Source: CAD feature listing. Evaluate the final solid. Frame: model axes, mm. A direction names the side the tool comes from. Give positions to 0.01 mm unless a question says otherwise; leave off trailing zeros. Order: outer loops, then holes, each group sorted by start corner. A loop starts at its lowest first (then second) coordinate and runs counter-clockwise, first axis right, second up.
Autodesk Inventor part; units mm, degrees
ref_plane "YZ Plane" through (0, 0, 0) normal (1, 0, 0) x (0, 1, 0)
ref_plane "XZ Plane" through (0, 0, 0) normal (0, 1, 0) x (-1, 0, 0)
ref_plane "XY Plane" through (0, 0, 0) normal (0, 0, 1) x (1, 0, 0)
sketch "Sketch1" plane through (0, 0, 0) normal (0, 1, 0) x (-1, 0, 0)
  circle A0 centre (0, 0) radius 55
  circle A1 centre (0, 0) radius 2.6
  dimension "d0" = 110
  dimension "d1" = 5.2
extrude "Extrusion1" add sketch "Sketch1" along normal blind 5
sketch "Sketch2" plane through (0, 5, 0) normal (0, 1, 0) x (1, 0, 0)
  point P0 (0, 0)
sketch "Sketch4" plane through (0, 5, 0) normal (0, 1, 0) x (1, 0, 0)
  circle A0 centre (0, 0) radius 21.9076
  circle A1 centre (0, 0) radius 35
  circle A2 centre (-35, 0) radius 15.2
  circle A3 centre (-17.5, -30.3109) radius 15.2
  circle A4 centre (17.5, -30.3109) radius 15.2
  circle A5 centre (35, 0) radius 15.2
  circle A6 centre (17.5, 30.3109) radius 15.2
  circle A7 centre (-17.5, 30.3109) radius 15.2
  circle A8 centre (-21.9076, 0) radius 5.15
  circle A9 centre (-15.491, -15.491) radius 5.15
  circle A10 centre (0, -21.9076) radius 5.15
  circle A11 centre (15.491, -15.491) radius 5.15
  circle A12 centre (21.9076, 0) radius 5.15
  circle A13 centre (15.491, 15.491) radius 5.15
  circle A14 centre (0, 21.9076) radius 5.15
  circle A15 centre (-15.491, 15.491) radius 5.15
  dimension "d13" = 70
  dimension "d8" = 30.4
  dimension "d11" = 360
  dimension "d14" = 10.3
  dimension "d17" = 360
extrude "Extrusion3" cut sketch "Sketch4" against normal blind 5 contours A0 A12 A5 | A0 A12 | A12 A5 A0 | A0 A5 A1 A12 | A0 A5 A12 | A5 A1 | A6 A13 A0 | A0 A13 A6 | A6 A0 A13 | A13 A0 A6 A14 A1 | A1 A6 | A4 A11 A0 | A0 A11 A4 | A4 A1 A10 A0 A11 | A11 A0 A4 | A4 A1 | A6 A14 | A7 A14 A0 A15 A1 | A1 A7 | A10 A4 | A3 A1 | A1 A3 A9 A0 A10 | A7 A14 | A10 A3 | A7 A15 A0 | A2 A0 A8 A1 | A1 A2 | A15 A0 A7 | A0 A9 A3 | A3 A0 A9 | A15 A7 A0 | A2 A8 A0 | A0 A3 A9 | A0 A8 A2 | A8 A2 A0 | A0 A8 picked at (11.9722, 17.0625) picked at (16.7139, 17.1312) picked at (8.2786, 19.0961) picked at (16.7139, -17.1312) picked at (11.9722, -17.0625) picked at (8.2786, -19.0961) picked at (-8.2786, 19.0961) picked at (-16.7226, 17.1255) picked at (-8.2786, -19.0961) picked at (-16.7226, -17.1255) picked at (-11.9722, 17.0625) picked at (-11.9722, -17.0625)
sketch "Sketch5" plane through (0, 5, 0) normal (0, 1, 0) x (1, 0, 0)
  point P0 (0, 0)
sketch "Sketch6" plane through (0, 0, 0) normal (0, -1, 0) x (1, 0, 0)
  circle A0 centre (0, 0) radius 55
extrude "Extrusion4" add sketch "Sketch6" along normal blind 0.5
sketch "Sketch7" plane through (0, 5, 0) normal (0, 1, 0) x (1, 0, 0)
  circle A0 centre (-35, 0) radius 15.2
  circle A1 centre (-35, 0) radius 12.5
  circle A2 centre (-17.5, -30.3109) radius 15.2
  circle A3 centre (-17.5, -30.3109) radius 12.5
  circle A4 centre (17.5, -30.3109) radius 15.2
  circle A5 centre (17.5, -30.3109) radius 12.5
  circle A6 centre (35, 0) radius 15.2
  circle A7 centre (35, 0) radius 12.5
  circle A8 centre (17.5, 30.3109) radius 15.2
  circle A9 centre (17.5, 30.3109) radius 12.5
  circle A10 centre (-17.5, 30.3109) radius 15.2
  circle A11 centre (-17.5, 30.3109) radius 12.5
  point P0 (0, 0)
  dimension "d23" = 25
  dimension "d24" = 25
  dimension "d25" = 25
  dimension "d26" = 25
  dimension "d27" = 25
  dimension "d28" = 25
extrude "Extrusion5" cut sketch "Sketch7" against normal blind 86.25 contours A1 | A3 | A5 | A7 | A9 | A11
sketch "Sketch8" plane through (0, 5, 0) normal (0, 1, 0) x (1, 0, 0)
  circle A0 centre (0, 0) radius 2.6
extrude "Extrusion6" cut sketch "Sketch8" against normal blind 86.25
sketch "Sketch9" plane through (0, 5, 0) normal (0, 1, 0) x (1, 0, 0)
  circle A0 centre (17.5, 30.3109) radius 15.2
  arc A1 (26.25, 15.1554) -> (0, 30.3109) centre (17.5, 30.3109) ccw
  circle A2 centre (35, 0) radius 15.2
  arc A3 (26.25, -15.1554) -> (26.25, 15.1554) centre (35, 0) ccw
  circle A4 centre (17.5, -30.3109) radius 15.2
  arc A5 (0, -30.3109) -> (26.25, -15.1554) centre (17.5, -30.3109) ccw
  circle A6 centre (-17.5, -30.3109) radius 15.2
  arc A7 (-26.25, -15.1554) -> (0, -30.3109) centre (-17.5, -30.3109) ccw
  circle A8 centre (-35, 0) radius 15.2
  arc A9 (-26.25, 15.1554) -> (-26.25, -15.1554) centre (-35, 0) ccw
  circle A10 centre (-17.5, 30.3109) radius 15.2
  arc A11 (0, 30.3109) -> (-26.25, 15.1554) centre (-17.5, 30.3109) ccw
  circle A12 centre (0, 0) radius 2.6
  circle A13 centre (0, 0) radius 65.8368
  dimension "d33" = 35
  dimension "d34" = 35
  dimension "d35" = 35
  dimension "d36" = 35
  dimension "d37" = 35
  dimension "d38" = 35
  dimension "d39" = 131.6736
extrude "Extrusion7" cut sketch "Sketch9" against normal blind 86.25 contours A13
properties part number "generator 12smaller"
1) Section query C-C, the plane y = 3.85. Return the cut outline in (x, z).
Report:
outline: (-26.25, -15.16) arc R17.5 ccw (long way) to (0, -30.31) arc R17.5 ccw (long way) to (26.25, -15.16) arc R17.5 ccw (long way) to (26.25, 15.16) arc R17.5 ccw (long way) to (0, 30.31) arc R17.5 ccw (long way) to (-26.25, 15.16) arc R17.5 ccw (long way) to start; hole circle Ø30.4 at (-35, 0); hole circle Ø30.4 at (-17.5, -30.31); hole circle Ø30.4 at (-17.5, 30.31); hole circle Ø5.2 at (0, 0); hole circle Ø30.4 at (17.5, -30.31); hole circle Ø30.4 at (17.5, 30.31); hole circle Ø30.4 at (35, 0)
2) Draft query along X for faces 1 (the flat face through (-4, 5, -3)), 2 (the cylindrical face through (-27.42, -0.247, 37.917)). Return one class per face: +X half, -X half, draft (parallel to the pull), parting line (faces both ways), or undercut.
Report:
face 1: draft
face 2: undercut
3) Reachability of faces 3 (the cylindrical face through (23.27, -0.25, 41.4)), 4 (the cylindrical face through (-50.185, 2.535, -0.668)) from +Z, -Z, +X, -X, +Y, -Y: full face, straight path, thin tool, end or side. Return the list, or none.
Report:
face 3: +Y, -Y
face 4: +Y
4) Pin query (flat end, axial travel): pin 1 (15 mm diameter, centred on x = 20.5, z = 25.5, fed in from +Y); pin 2 (10 mm diameter, centred on x = 2.5, z = -28.5, fed in from +Y); pin 3 (1 mm diameter, centred on y = 3.5, z = -3, fed in from +X). Return the tip coordinate at first contact, or that it passes through.
Report:
pin 1: stops at y = 0
pin 2: stops at y = 5
pin 3: stops at x = 52.32
5) Material intervals for L1, parallel to Z at x = 17.5, y = -0.3; L2, parallel to X at y = 0.3, z = 29.5; L3, parallel to X at y = 3.05, z = 14, sorted ascending.
Report:
L1: z = -47.81 to -42.81, -17.81 to 17.81, 42.81 to 47.81
L2: x = -34.98 to -32.68, -2.32 to 2.32, 32.68 to 34.98
L3: x = -45.5 to -40.92, -29.08 to 29.08, 40.92 to 45.5
6) Section query B-B, the plane z = 39.5. Return the cut outline in (x, y), and give its area (3 significant figures).
Report:
outline: (-32.39, -0.5) - (-25.97, -0.5) - (-25.97, 0) - (-29.61, 0) - (-29.61, 5) - (-32.39, 5) - close; (-9.03, -0.5) - (-2.61, -0.5) - (-2.61, 5) - (-5.39, 5) - (-5.39, 0) - (-9.03, 0) - close; (2.61, -0.5) - (9.03, -0.5) - (9.03, 0) - (5.39, 0) - (5.39, 5) - (2.61, 5) - close; (25.97, -0.5) - (32.39, -0.5) - (32.39, 5) - (29.61, 5) - (29.61, 0) - (25.97, 0) - close
area: 68.5 mm2
7) Section query A-A, the plane x = -17.5. Return the cut outline in (y, z), and give its area (3 significant figures).
Report:
outline: (-0.5, -47.81) - (5, -47.81) - (5, -45.51) - (0, -45.51) - (0, -42.81) - (-0.5, -42.81) - close; (-0.5, -17.81) - (0, -17.81) - (0, -15.11) - (5, -15.11) - (5, 15.11) - (0, 15.11) - (0, 17.81) - (-0.5, 17.81) - close; (-0.5, 42.81) - (0, 42.81) - (0, 45.51) - (5, 45.51) - (5, 47.81) - (-0.5, 47.81) - close
area: 197 mm2
8) Section query D-D, the plane z = 21.5. Return the cut outline in (x, y), and give its area (3 significant figures).
Report:
outline: (-32.62, -0.5) - (-26.37, -0.5) - (-26.37, 0) - (-29.89, 0) - (-29.89, 5) - (-32.62, 5) - close; (-8.63, -0.5) - (8.63, -0.5) - (8.63, 0) - (5.11, 0) - (5.11, 5) - (-5.11, 5) - (-5.11, 0) - (-8.63, 0) - close; (26.37, -0.5) - (32.62, -0.5) - (32.62, 5) - (29.89, 5) - (29.89, 0) - (26.37, 0) - close
area: 93.4 mm2
